Input: part model. Units: mm. Frame: model coordinates. A direction names the side the tool comes from. Coordinates: 2 decimals unless noted, no trailing zeros. Write each loop counter-clockwise with the first axis right and the second up, starting at its lowest first coordinate (ties: lowest second). Pieces come first, ordered by that corner, then holes. Notation, with made-up numbers: (15, 78) - (54, 78) arc R9 cw to (54, 87) - close; hole circle Ø7 at (55, 63). An arc over 180 degrees is marked (long way). Put each result on its own line as item: value. Start each with the question number.
1. Cut plane C-C, the plane y = 253.5. Return loops of the section in (x, z).
2. Pin query (flat end, axial travel): pin 1 (10 mm diameter, centred on x = 152, y = 253, fed in from -Z); pin 2 (5.5 mm diameter, centred on x = 104.5, y = 255.5, fed in from +Z); pin 3 (3 mm diameter, centred on y = 265, z = 13, fed in from -X); pin 4 (1.8 mm diameter, centred on x = 202.5, y = 139, fed in from -Z). Return the tip coordinate at first contact, or that it passes through.
3. Pull-direction query (Y, two-part tool) for faces 1 (the flat face through (141, 292.5, 4)), 2 (the flat face through (80, 216, 2)), 3 (the flat face through (107, 126, 15)); classes: released by +Y, released by -Y, zero draft, split by the parting line, or undercut.
4. Line query: line 1 (Y direction, x = 47.5, z = 32); line 2 (X direction, y = 23.5, z = 5.5). Output: solid intervals per line, ascending.
5. Cut plane A-A, the plane z = 32.5. Return loops of the section in (x, y).
6. Cut plane D-D, the plane y = 37.5. Return loops of the section in (x, z), and give its area (3 significant figures).
7. Cut plane B-B, the plane x = 23. Return loops of the section in (y, z).
8. Access query for faces 4 (the flat face through (140, 29, 4)), 5 (the flat face through (40, 8, 37)), 6 (the flat face through (204, 107, 2)). Directions: +Z, -Z, +X, -X, +Y, -Y. A direction counts if a zero-diameter tool reaches every point of the face in a straight line with its end or side. Return the directions, or none.
from build123d import *

# Parameters (mm, degrees)
EXTRUDE_1_DEPTH         = 8
CUT_EXTRUDE_1_DEPTH     = 2
SKETCH_3_R              = 2
CUT_EXTRUDE_2_DEPTH     = 5
SKETCH_4_W              = 62
SKETCH_4_H              = 8
EXTRUDE_2_DEPTH         = 60
FILLET_1_R              = 2
SKETCH_5_W              = 5
SKETCH_5_H              = 20
SKETCH_5_W_2            = 15
SKETCH_5_H_2            = 5
SKETCH_5_H_3            = 15
EXTRUDE_4_DEPTH         = 7
SKETCH_6_W              = 45
SKETCH_6_H              = 8
CUT_EXTRUDE_3_DEPTH     = 366.042805709
CUT_EXTRUDE_START       = -8
CUT_EXTRUDE_4_OUTLINE_W = 70
CUT_EXTRUDE_4_OUTLINE_H = 24.5
CUT_EXTRUDE_4_DEPTH     = 8
CUT_EXTRUDE_4_2_DEPTH   = 7
CUT_EXTRUDE_4_3_DEPTH   = 7


# Read off the part's stored shape, not the designer's step: 컷-돌출4
with BuildPart() as part:
    # 스케치1 → 보스-돌출1 (new body)
    with BuildSketch(Plane.XY):
        Polygon((0, 0), (140, 0), (140, 97.5), (210, 97.5), (210, 292.5), (70, 292.5), (70, 195), (0, 195), align=None)
    extrude(amount=EXTRUDE_1_DEPTH)

    # 스케치2 → 컷-돌출1 (cut)
    with BuildSketch(Plane.XY):
        Polygon((200.25, 287.531088913), (198.5, 284.5), (200.25, 281.468911087), (203.75, 281.468911087), (205.5, 284.5), (203.75, 287.531088913), align=None)
        Polygon((76.25, 287.531088913), (74.5, 284.5), (76.25, 281.468911087), (79.75, 281.468911087), (81.5, 284.5), (79.75, 287.531088913), align=None)
        Polygon((6.25, 189.986613874), (4.5, 186.955524961), (6.224322324, 183.968911087), (9.775677676, 183.968911087), (11.5, 186.955524961), (9.75, 189.986613874), align=None)
        Polygon((76.25, 217.531088913), (74.5, 214.5), (76.25, 211.468911087), (79.75, 211.468911087), (81.5, 214.5), (79.75, 217.531088913), align=None)
        Polygon((200.25, 140.531088913), (198.5, 137.5), (200.25, 134.468911087), (203.75, 134.468911087), (205.5, 137.5), (203.75, 140.531088913), align=None)
        Polygon((200.25, 108.531088913), (198.5, 105.5), (200.25, 102.468911087), (203.75, 102.468911087), (205.5, 105.5), (203.75, 108.531088913), align=None)
        Polygon((144.5, 105.5), (146.25, 102.468911087), (149.75, 102.468911087), (151.5, 105.5), (149.75, 108.531088913), (146.25, 108.531088913), align=None)
        Polygon((14.25, 102.531088913), (12.5, 99.5), (14.25, 96.468911087), (17.75, 96.468911087), (19.5, 99.5), (17.75, 102.531088913), align=None)
    extrude(amount=CUT_EXTRUDE_1_DEPTH, mode=Mode.SUBTRACT)

    # 스케치3 → 컷-돌출2 (cut)
    with BuildSketch(Plane(origin=(0, 0, 2), x_dir=(-1, 0, 0), z_dir=(0, 0, -1))):
        with Locations((-202.01036292, 284.501088913)):
            Circle(SKETCH_3_R)
        with Locations((-78.01036292, 284.501088913)):
            Circle(SKETCH_3_R)
        with Locations((-78.01036292, 214.498911087)):
            Circle(SKETCH_3_R)
        with Locations((-8.01036292, 186.998911087)):
            Circle(SKETCH_3_R)
        with Locations((-201.989637708, 137.501088913)):
            Circle(SKETCH_3_R)
        with Locations((-202.011036292, 105.501088913)):
            Circle(SKETCH_3_R)
        with Locations((-148.01036292, 105.501088913)):
            Circle(SKETCH_3_R)
        with Locations((-16.01036292, 99.528088913)):
            Circle(SKETCH_3_R)
    extrude(amount=-CUT_EXTRUDE_2_DEPTH, mode=Mode.SUBTRACT)

    # 스케치4 → 보스-돌출2 (add)
    with BuildSketch(Plane.XY.offset(8)):
        Polygon((0, 97.5), (0, 0), (8, 0), (8, 8), (8, 97.5), align=None)
        with Locations((39, 4)):
            Rectangle(SKETCH_4_W, SKETCH_4_H)
    extrude(amount=EXTRUDE_2_DEPTH)

    # 필렛1
    fillet_1_edges = [part.edges().sort_by_distance(p)[0] for p in [
        (0, 0, 34),
        (105, 0, 8),
        (70, 0, 38),
        (8, 8, 38),
        (0, 97.5, 38),
        (35, 0, 68),
        (39, 8, 68),
        (8, 52.75, 68),
        (0, 48.75, 68),
        (0, 146.25, 8),
    ]]
    fillet(fillet_1_edges, radius=FILLET_1_R)

    # 스케치5 → 보스-돌출4 (add)
    with BuildSketch(Plane.XY.offset(8)):
        with Locations((104.5, 257.5)):
            Rectangle(SKETCH_5_W, SKETCH_5_H)
        with Locations((165.5, 265)):
            Rectangle(SKETCH_5_W_2, SKETCH_5_H_2)
        Polygon((173, 267.5), (173, 262.5), (173, 247.5), (178, 247.5), (178, 267.5), align=None)
        Polygon((122, 127.5), (107, 127.5), (102, 127.5), (102, 122.5), (122, 122.5), align=None)
        with Locations((104.5, 135)):
            Rectangle(SKETCH_5_W, SKETCH_5_H_3)
        with Locations((165.5, 125)):
            Rectangle(SKETCH_5_W_2, SKETCH_5_H_2)
        Polygon((173, 142.5), (173, 127.5), (173, 122.5), (178, 122.5), (178, 142.5), align=None)
    extrude(amount=EXTRUDE_4_DEPTH)

    # 스케치6 → 컷-돌출3 (cut, through all)
    with BuildSketch(Plane.XY.offset(8)):
        with Locations((129.5, 271.5)):
            Rectangle(SKETCH_6_W, SKETCH_6_H)
    extrude(amount=-CUT_EXTRUDE_3_DEPTH, mode=Mode.SUBTRACT)

    # 컷-돌출4 outline → 컷-돌출4 (cut)
    with BuildSketch(Plane.XY.offset(8).offset(CUT_EXTRUDE_START)):
        with Locations((105, 70.25)):
            Rectangle(CUT_EXTRUDE_4_OUTLINE_W, CUT_EXTRUDE_4_OUTLINE_H)
    extrude(amount=CUT_EXTRUDE_4_DEPTH, mode=Mode.SUBTRACT)

    # Cut-Extrude 4 2 outline → Cut-Extrude 4 2 (cut)
    with BuildSketch(Plane.XY.offset(8)):
        with BuildLine():
            Line((173, 142.5), (173, 141.5))
            ThreePointArc((173, 141.5), (173.292893219, 142.207106781), (174, 142.5))
            Line((174, 142.5), (173, 142.5))
        make_face()
        with BuildLine():
            Line((178, 142.5), (177, 142.5))
            ThreePointArc((177, 142.5), (177.707106781, 142.207106781), (178, 141.5))
            Line((178, 141.5), (178, 142.5))
        make_face()
        with BuildLine():
            Line((178, 122.5), (178, 123.5))
            ThreePointArc((178, 123.5), (177.707106781, 122.792893219), (177, 122.5))
            Line((177, 122.5), (178, 122.5))
        make_face()
        with BuildLine():
            ThreePointArc((159, 122.5), (158.292893219, 122.792893219), (158, 123.5))
            Line((158, 123.5), (158, 122.5))
            Line((158, 122.5), (159, 122.5))
        make_face()
        with BuildLine():
            Line((107, 142.5), (106, 142.5))
            ThreePointArc((106, 142.5), (106.707106781, 142.207106781), (107, 141.5))
            Line((107, 141.5), (107, 142.5))
        make_face()
        with BuildLine():
            ThreePointArc((102, 141.5), (102.292893219, 142.207106781), (103, 142.5))
            Line((103, 142.5), (102, 142.5))
            Line((102, 142.5), (102, 141.5))
        make_face()
        with BuildLine():
            ThreePointArc((103, 122.5), (102.292893219, 122.792893219), (102, 123.5))
            Line((102, 123.5), (102, 122.5))
            Line((102, 122.5), (103, 122.5))
        make_face()
        with BuildLine():
            Line((122, 122.5), (122, 123.5))
            ThreePointArc((122, 123.5), (121.707106781, 122.792893219), (121, 122.5))
            Line((121, 122.5), (122, 122.5))
        make_face()
        with BuildLine():
            Line((107, 247.5), (107, 248.5))
            ThreePointArc((107, 248.5), (106.707106781, 247.792893219), (106, 247.5))
            Line((106, 247.5), (107, 247.5))
        make_face()
        with BuildLine():
            Line((102, 247.5), (103, 247.5))
            ThreePointArc((103, 247.5), (102.292893219, 247.792893219), (102, 248.5))
            Line((102, 248.5), (102, 247.5))
        make_face()
        with BuildLine():
            ThreePointArc((102, 266.5), (102.292893219, 267.207106781), (103, 267.5))
            Line((103, 267.5), (102, 267.5))
            Line((102, 267.5), (102, 266.5))
        make_face()
        with BuildLine():
            ThreePointArc((174, 247.5), (173.292893219, 247.792893219), (173, 248.5))
            Line((173, 248.5), (173, 247.5))
            Line((173, 247.5), (174, 247.5))
        make_face()
        with BuildLine():
            ThreePointArc((178, 248.5), (177.707106781, 247.792893219), (177, 247.5))
            Line((177, 247.5), (178, 247.5))
            Line((178, 247.5), (178, 248.5))
        make_face()
        with BuildLine():
            ThreePointArc((177, 267.5), (177.707106781, 267.207106781), (178, 266.5))
            Line((178, 266.5), (178, 267.5))
            Line((178, 267.5), (177, 267.5))
        make_face()
        with BuildLine():
            Line((158, 267.5), (158, 266.5))
            ThreePointArc((158, 266.5), (158.292893219, 267.207106781), (159, 267.5))
            Line((159, 267.5), (158, 267.5))
        make_face()
    extrude(amount=CUT_EXTRUDE_4_2_DEPTH, mode=Mode.SUBTRACT)

    # Cut-Extrude 4 3 outline → Cut-Extrude 4 3 (add)
    with BuildSketch(Plane.XY.offset(8)):
        with BuildLine():
            Line((173, 127.5), (173, 128.5))
            ThreePointArc((173, 128.5), (172.707106781, 127.792893219), (172, 127.5))
            Line((172, 127.5), (173, 127.5))
        make_face()
        with BuildLine():
            ThreePointArc((108, 127.5), (107.292893219, 127.792893219), (107, 128.5))
            Line((107, 128.5), (107, 127.5))
            Line((107, 127.5), (108, 127.5))
        make_face()
        with BuildLine():
            ThreePointArc((172, 262.5), (172.707106781, 262.207106781), (173, 261.5))
            Line((173, 261.5), (173, 262.5))
            Line((173, 262.5), (172, 262.5))
        make_face()
    extrude(amount=CUT_EXTRUDE_4_3_DEPTH)


solid = part.part
Report:
1. outline: (70, 0) - (210, 0) - (210, 8) - (178, 8) - (178, 15) - (173, 15) - (173, 8) - (107, 8) - (107, 15) - (102, 15) - (102, 8) - (70, 8) - close
2. pin 1: stops at z = 0
2. pin 2: stops at z = 15
2. pin 3: stops at x = 102
2. pin 4: stops at z = 2
3. face 1: released by +Y
3. face 2: undercut
3. face 3: zero draft
4. line 1: y = 0 to 8
4. line 2: x = 0 to 140
5. outline: (0, 2) arc R2 ccw to (2, 0) - (68, 0) arc R2 ccw to (70, 2) - (70, 8) - (10, 8) arc R2 cw to (8, 10) - (8, 97.5) - (2, 97.5) arc R2 ccw to (0, 95.5) - close
6. outline: (0, 0) - (140, 0) - (140, 8) - (8, 8) - (8, 66) arc R2 ccw to (6, 68) - (2, 68) arc R2 ccw to (0, 66) - close
6. area: 1,600 mm^2
7. outline: (0, 0) - (195, 0) - (195, 8) - (8, 8) - (8, 66) arc R2 ccw to (6, 68) - (2, 68) arc R2 ccw to (0, 66) - close
8. face 4: +Z, -Z, +X, -Y
8. face 5: +Z, +X, +Y
8. face 6: -Z
